from build123d import *

# Parameters (mm, degrees)
F0_W     = 73
F0_H     = 78
F0_W_2   = 112
F0_H_2   = 35
F1_DEPTH = 5
F2_R     = 5
F3_R     = 5
F6_D     = 4.1
F8_D     = 43
F9_D     = 11


with BuildPart() as f1:
    # F0 (on Top) → F1 (new body)
    with BuildSketch(Plane.XY):
        Polygon((-56, 50), (-86, 50), (-272.5, -15), (-272.5, -50), (-199.5, -50), (199.5, -50), (272.5, -50), (272.5, -15), (86, 50), (56, 50), align=None)
        with Locations((-236, -89)):
            Rectangle(F0_W, F0_H)
        with Locations((236, -89)):
            Rectangle(F0_W, F0_H)
        with Locations((0, 67.5)):
            Rectangle(F0_W_2, F0_H_2)
    extrude(amount=F1_DEPTH)

    # F2
    f2_edges = [f1.edges().sort_by_distance(p)[0] for p in [
        (-272.5, -128, 2.5),
        (-199.5, -128, 2.5),
        (199.5, -128, 2.5),
        (272.5, -128, 2.5),
        (272.5, -15, 2.5),
        (-272.5, -15, 2.5),
        (-199.5, -50, 2.5),
        (199.5, -50, 2.5),
        (-56, 50, 2.5),
        (-56, 85, 2.5),
        (56, 85, 2.5),
        (56, 50, 2.5),
    ]]
    fillet(f2_edges, radius=F2_R)

    # F3
    f3_edges = [f1.edges().sort_by_distance(p)[0] for p in [
        (86, 50, 2.5),
        (-86, 50, 2.5),
    ]]
    fillet(f3_edges, radius=F3_R)

    # F6 (through all)
    with Locations(Plane(origin=(0, 0, 0), x_dir=(1, 0, 0), z_dir=(0, 0, -1))):
        with Locations((-31, -17.5), (31, -17.5)):
            Hole(F6_D / 2)

    # F8 (through all)
    with Locations(Plane(origin=(0, 0, 0), x_dir=(1, 0, 0), z_dir=(0, 0, -1))):
        with Locations((-236, 94), (236, 94)):
            Hole(F8_D / 2)

    # F9 (through all)
    with Locations(Plane(origin=(0, 0, 0), x_dir=(1, 0, 0), z_dir=(0, 0, -1))):
        with Locations((-36, -68.5), (36, -68.5), (0, 33.5)):
            Hole(F9_D / 2)


solid = f1.part
Can you work these out from the model? Positions are in its coordinate system, mm. Round coordinates to 2 decimals unless told otherwise and drop trailing zeros. Order: outer loops, then holes, each group sorted by start corner. A loop starts at its lowest first (then second) coordinate and runs counter-clockwise, first axis right, second up. Notation, with made-up numbers: (88.5, -10.75) - (136.5, -10.75) arc R23 cw to (136.5, -2.75) - close; hole circle Ø3 at (28.5, -17). An arc over 180 degrees is marked (long way). Answer in a Markdown table with one row per item.
(1) Suppose I cut it at B-B, the plane y = -94. Please give me the cut outline in (x, z).
From the geometry:
| item | result |
|---|---|
| outline | (-272.5, 0) - (-257.5, 0) - (-257.5, 5) - (-272.5, 5) - close; (-214.5, 0) - (-199.5, 0) - (-199.5, 5) - (-214.5, 5) - close; (199.5, 0) - (214.5, 0) - (214.5, 5) - (199.5, 5) - close; (257.5, 0) - (272.5, 0) - (272.5, 5) - (257.5, 5) - close |
(2) Suppose I cut it at A-A, the plane x = -236. Please give me the cut outline in (y, z), plus the area to 3 significant figures.
From the geometry:
| item | result |
|---|---|
| outline | (-128, 0) - (-115.5, 0) - (-115.5, 5) - (-128, 5) - close; (-72.5, 0) - (-2.28, 0) - (-2.28, 5) - (-72.5, 5) - close |
| area | 414 mm2 |
(3) For P1, Ø3.5, axis at x = 31, y = 17.5, coming from the -Z side; P2, Ø2.5, axis at x = 69.5, z = 2.5, coming from the +Y side; P3, Ø6.5, axis at x = -31, y = 17.5, coming from the +Z side; P4, Ø2.5, axis at y = 63, z = 3, coming from the +X side, each with a flat end and sliding along its axis, tell me the tip position at first contact or that it passes through.
From the geometry:
| item | result |
|---|---|
| P1 | passes through |
| P2 | stops at y = 50 |
| P3 | stops at z = 5 |
| P4 | stops at x = 56 |
(4) Suppose I cut it at D-D, the plane x = 0. Please give me the cut outline in (y, z).
From the geometry:
| item | result |
|---|---|
| outline | (-50, 0) - (-39, 0) - (-39, 5) - (-50, 5) - close; (-28, 0) - (85, 0) - (85, 5) - (-28, 5) - close |
(5) Please list where these lines run through material, in increasing order: L1, parallel to X at y = 68.5, z = 2.85; L2, parallel to X at y = -94, z = 2.9; L3, parallel to X at y = -33.5, z = 3.45. Write a range as from..to.
From the geometry:
| item | result |
|---|---|
| L1 | x = -56..-41.5, -30.5..30.5, 41.5..56 |
| L2 | x = -272.5..-257.5, -214.5..-199.5, 199.5..214.5, 257.5..272.5 |
| L3 | x = -272.5..-5.5, 5.5..272.5 |
(6) If we mould it in two halves opening along X, with no side actions, what happens to faces 1 (the face through (-256.507, -100.458, 2.535)), 2 (the face through (0.716, -38.953, 2.535)), 3 (the face through (-176.7, 18.39, 2.46)), 4 (the face through (-4, -20, 5))? For each: released by +X, released by -X, zero draft, split by the parting line, or undercut.
From the geometry:
| item | result |
|---|---|
| face 1 | undercut |
| face 2 | undercut |
| face 3 | released by -X |
| face 4 | zero draft |
(7) Suppose I cut it at C-C, the plane z = 2.65. Count the separate pieces of the cut face and the enclosed holes in it, plus the area to 3 significant figures.
From the geometry:
| item | result |
|---|---|
| separate pieces | 1 |
| enclosed holes | 7 |
| area | 54,500 mm2 |
